For this review, take the finished solid that the model builds, in its own axes (mm). Face numbers are marked on the shaded views. Give positions to 0.01 mm unless a question says otherwise; leave off trailing zeros. Loops run counter-clockwise (first coordinate to the right, second up) from the corner with the lowest first, then second, coordinate; pieces in that order, holes last.
```python
from build123d import *

# Parameters (mm, degrees)
BOSS_EXTRUDE2_DEPTH = 30
CUT_EXTRUDE1_DEPTH  = 125
SKETCH4_W           = 125
SKETCH4_H           = 2
SKETCH4_H_2         = 2.5
BOSS_EXTRUDE4_DEPTH = 2.5
SKETCH5_W           = 125
SKETCH5_H           = 2.5
SKETCH5_H_2         = 2
BOSS_EXTRUDE5_DEPTH = 2.5
SKETCH6_R           = 2
CUT_EXTRUDE2_DEPTH  = 20


with BuildPart() as part:
    # Sketch1 → Boss-Extrude2 (new body)
    with BuildSketch(Plane(origin=(0, 0, 0), x_dir=(1, 0, 0), z_dir=(0, 1, 0))):
        Polygon((-5, 130), (-5, 0), (0, 0), (65, 0), (65, 130), align=None)
    extrude(amount=BOSS_EXTRUDE2_DEPTH)

    # Sketch3 → Cut-Extrude1 (cut)
    with BuildSketch(Plane.XY):
        Polygon((24.738126678, 25), (0, 25), (0, 5), (60, 5), (60, 25), align=None)
    extrude(amount=-CUT_EXTRUDE1_DEPTH, mode=Mode.SUBTRACT)

    # Sketch4 → Boss-Extrude4 (add)
    with BuildSketch(Plane(origin=(0, 0, 0), x_dir=(0, 0, -1), z_dir=(1, 0, 0))):
        with Locations((62.5, 11.5)):
            Rectangle(SKETCH4_W, SKETCH4_H)
        with Locations((62.5, 6.25)):
            Rectangle(SKETCH4_W, SKETCH4_H_2)
    extrude(amount=BOSS_EXTRUDE4_DEPTH)

    # Sketch5 → Boss-Extrude5 (add)
    with BuildSketch(Plane.ZY.offset(-60)):
        with Locations((-62.5, 6.25)):
            Rectangle(SKETCH5_W, SKETCH5_H)
        with Locations((-62.5, 11.5)):
            Rectangle(SKETCH5_W, SKETCH5_H_2)
    extrude(amount=BOSS_EXTRUDE5_DEPTH)

    # Sketch6 → Cut-Extrude2 (cut)
    with BuildSketch(Plane.XY):
        with Locations((-2.171572875, 27.171572875)):
            Circle(SKETCH6_R)
        with Locations((62.171572875, 27.171572875)):
            Circle(SKETCH6_R)
        with Locations((62.171572875, 2.828427125)):
            Circle(SKETCH6_R)
        with Locations((-2.171572875, 2.828427125)):
            Circle(SKETCH6_R)
    extrude(amount=-CUT_EXTRUDE2_DEPTH, mode=Mode.SUBTRACT)


solid = part.part
```
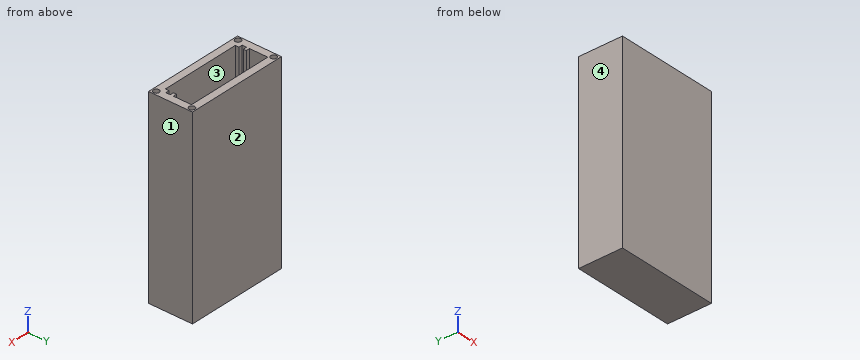
Q1. Consider section A-A on z = -52.5. Give the boundary of the cut face in (x, y), plus the area to 4 significant figures.
Answers:
outline: (-5, 0) - (65, 0) - (65, 30) - (-5, 30) - close; hole (0, 7.5) - (2.5, 7.5) - (2.5, 5) - (57.5, 5) - (57.5, 7.5) - (60, 7.5) - (60, 10.5) - (57.5, 10.5) - (57.5, 12.5) - (60, 12.5) - (60, 25) - (0, 25) - (0, 12.5) - (2.5, 12.5) - (2.5, 10.5) - (0, 10.5) - close
area: 922.5 mm2
Q2. Consider section C-C on x = 54.5. Give the boundary of the cut face in (y, z).
Answers:
outline: (0, -130) - (30, -130) - (30, 0) - (25, 0) - (25, -125) - (5, -125) - (5, 0) - (0, 0) - close
Q3. Mouldability with a two-part tool opening along X and no side actions: class the marked faces 1, 2, 3 and 4 as +X half, -X half, draft (parallel to the pull), parting line (faces both ways), or undercut.
Answers:
face 1: +X half
face 2: draft
face 3: undercut
face 4: -X half
Q4. For pin 1 Ø10 at (x, y) = (29, 14.5) entering from +Z; pin 2 Ø4.5 at (x, y) = (62.17, 2.83) entering from +Z; pin 3 Ø3 at (x, y) = (62.17, 27.17) entering from +Z, all flat-tipped, find the tip position at first contact; note any pin that passes through.
Answers:
pin 1: stops at z = -125
pin 2: stops at z = 0
pin 3: stops at z = -20
Q5. For probe 1 along Y at (x, z) = (31, -72); probe 2 along X at (y, z) = (6.75, -5.5); probe 3 along X at (y, z) = (22.25, -49.5), list the stretches that pass through material, from the lowest coordinate up.
Answers:
probe 1: y = 0 to 5, 25 to 30
probe 2: x = -5 to 2.5, 57.5 to 65
probe 3: x = -5 to 0, 60 to 65
Q6. Consider section D-D on z = -13.5. Give the boundary of the cut face in (x, y), plus the area to 3 significant figures.
Answers:
outline: (-5, 0) - (65, 0) - (65, 30) - (-5, 30) - close; hole circle Ø4 at (-2.17, 2.83); hole circle Ø4 at (-2.17, 27.17); hole (0, 7.5) - (2.5, 7.5) - (2.5, 5) - (57.5, 5) - (57.5, 7.5) - (60, 7.5) - (60, 10.5) - (57.5, 10.5) - (57.5, 12.5) - (60, 12.5) - (60, 25) - (0, 25) - (0, 12.5) - (2.5, 12.5) - (2.5, 10.5) - (0, 10.5) - close; hole circle Ø4 at (62.17, 2.83); hole circle Ø4 at (62.17, 27.17)
area: 872 mm2
Q7. Consider section B-B on y = 16.75. Give the boundary of the cut face in (x, z), plus the area to 3 significant figures.
Answers:
outline: (-5, -130) - (65, -130) - (65, 0) - (60, 0) - (60, -125) - (0, -125) - (0, 0) - (-5, 0) - close
area: 1,600 mm2
